Geometry check sheet. Reference: the model listing, model coordinates, mm. Face numbers are marked on the shaded views. Give positions to 0.01 mm unless a question says otherwise; leave off trailing zeros. Write each loop counter-clockwise with the first axis right and the second up, starting at its lowest first coordinate (ties: lowest second). Pieces come first, ordered by that corner, then holes. Notation, with made-up numbers: (41.25, -2) - (77.25, -2) arc R15 cw to (77.25, 17) - close; hole circle Ø4 at (-4.5, 25.25). An arc over 180 degrees is marked (long way). Write item = value, one per line. Start each with the question number.
(1) Thickness scan on L1, parallel to X at y = -6.5, z = -2.5; L2, parallel to X at y = -5.25, z = -4; L3, parallel to Z at x = -16.5, y = -6. Record the ranges inside material, lowest first.
(2) Draft check along Z on the marked faces 1, 2, 3 and 4. Enter one of: pulls with the +Z half, pulls with the -Z half, needs draft (parallel to the pull), parting line crosses it, or undercut.
(3) Section check C-C, the plane x = 15. Enter the section's corners in (y, z), plus the area to 3 significant figures.
(4) Section check B-B, the plane y = -2. Enter the section's corners in (x, z), plus the area to 3 significant figures.
(5) Section check A-A, the plane x = -15. Enter the section's corners in (y, z), plus the area to 3 significant figures.
(6) Section check D-D, the plane z = -1.25. Give the number of separate pieces and of enclosed holes in the cut face, plus the area to 3 significant figures.
(7) Depth check by flat-ended pin: pin 1 Ø5.5 at (x, z) = (6.9, -2.68) entering from +Y; pin 2 Ø3.5 at (x, z) = (-0.95, -2.68) entering from -Y; pin 3 Ø5.5 at (x, z) = (-8.8, -2.68) entering from -Y. Enter the tip coordinate at first touch or a pass-through.
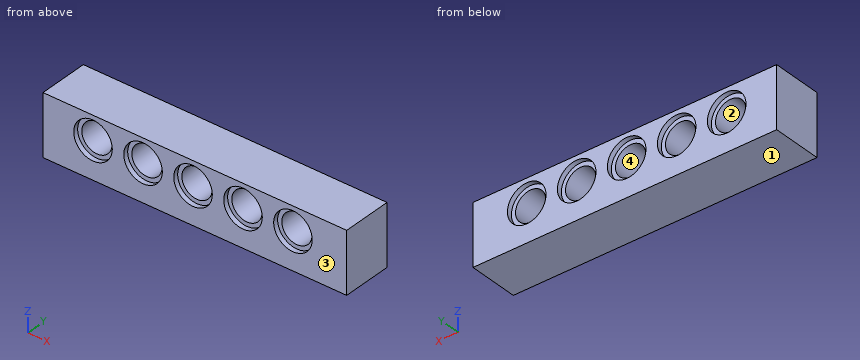
```python
from build123d import *

# Parameters (mm, degrees)
F0_W     = 47.7012
F0_H     = 9.5885
F1_DEPTH = 7.8232
F3_R     = 2.3749
F4_DEPTH = 8.12476
F5_R     = 3.02895
F5_R_2   = 3.028652
F6_DEPTH = 0.762
F7_R     = 3.02895
F7_R_2   = 3.028652
F8_DEPTH = 0.762


with BuildPart() as f1:
    # F0 (on Front) → F1 (new body)
    with BuildSketch(Plane.XZ):
        with Locations((-0.66396, -3.743826)):
            Rectangle(F0_W, F0_H)
    extrude(amount=F1_DEPTH)

    # F3 (on Front) → F4 (cut)
    with BuildSketch(Plane.XZ):
        with Locations((14.746952, -2.674865)):
            Circle(F3_R)
        with Locations((6.898352, -2.675486)):
            Circle(F3_R)
        with Locations((-0.950248, -2.676107)):
            Circle(F3_R)
        with Locations((-8.798848, -2.676728)):
            Circle(F3_R)
        with Locations((-16.65961, -2.677026)):
            Circle(F3_R)
    extrude(amount=F4_DEPTH, mode=Mode.SUBTRACT)

    # F5 (on Front) → F6 (cut)
    with BuildSketch(Plane.XZ):
        with Locations((14.746952, -2.674865)):
            Circle(F5_R)
        with Locations((6.898352, -2.675486)):
            Circle(F5_R)
        with Locations((-0.950248, -2.676107)):
            Circle(F5_R)
        with Locations((-8.798848, -2.676728)):
            Circle(F5_R_2)
        with Locations((-16.65961, -2.677026)):
            Circle(F5_R)
    extrude(amount=F6_DEPTH, mode=Mode.SUBTRACT)

    # F7 (on face) → F8 (cut)
    with BuildSketch(Plane.XZ.offset(7.8232)):
        with Locations((14.746952, -2.674865)):
            Circle(F7_R)
        with Locations((6.898352, -2.675486)):
            Circle(F7_R)
        with Locations((-0.950248, -2.676107)):
            Circle(F7_R)
        with Locations((-8.798848, -2.676728)):
            Circle(F7_R_2)
        with Locations((-16.65961, -2.677026)):
            Circle(F7_R)
    extrude(amount=-F8_DEPTH, mode=Mode.SUBTRACT)


solid = f1.part
```
Model answer:
q1.L1 = -24.51 to -19.03, -14.29 to -11.17, -6.43 to -3.32, 1.42 to 4.53, 9.27 to 12.38, 17.12 to 23.19
q1.L2 = -24.51 to -18.63, -14.69 to -10.77, -6.83 to -2.92, 1.02 to 4.93, 8.87 to 12.78, 16.72 to 23.19
q1.L3 = -8.54 to -5.05, -0.31 to 1.05
q2.face_1 = pulls with the -Z half
q2.face_2 = undercut
q2.face_3 = needs draft
q2.face_4 = undercut
q3.outline = (-7.82, -8.54) - (0, -8.54) - (0, -5.69) - (-0.76, -5.69) - (-0.76, -5.04) - (-7.06, -5.04) - (-7.06, -5.69) - (-7.82, -5.69) - close; (-7.82, 0.34) - (-7.06, 0.34) - (-7.06, -0.31) - (-0.76, -0.31) - (-0.76, 0.34) - (0, 0.34) - (0, 1.05) - (-7.82, 1.05) - close
q3.area = 36.1 mm²
q4.outline = (-24.51, -8.54) - (23.19, -8.54) - (23.19, 1.05) - (-24.51, 1.05) - close; hole circle Ø4.75 at (-16.66, -2.68); hole circle Ø4.75 at (-8.8, -2.68); hole circle Ø4.75 at (-0.95, -2.68); hole circle Ø4.75 at (6.9, -2.68); hole circle Ø4.75 at (14.75, -2.67)
q4.area = 369 mm²
q5.outline = (-7.82, -8.54) - (0, -8.54) - (0, -5.21) - (-0.76, -5.21) - (-0.76, -4.38) - (-7.06, -4.38) - (-7.06, -5.21) - (-7.82, -5.21) - close; (-7.82, -0.14) - (-7.06, -0.14) - (-7.06, -0.98) - (-0.76, -0.98) - (-0.76, -0.14) - (0, -0.14) - (0, 1.05) - (-7.82, 1.05) - close
q5.area = 45.9 mm²
q6.separate_pieces = 6
q6.enclosed_holes = 0
q6.area = 213 mm²
q7.pin_1 = -0.76
q7.pin_2 = through
q7.pin_3 = -7.06
